Part model, mm, in its own coordinate system. A direction names the side the tool comes from. Coordinates: 2 decimals unless noted, no trailing zeros. Loops run counter-clockwise (first coordinate to the right, second up) from the corner with the lowest first, then second, coordinate; pieces in that order, holes last. Notation, with made-up numbers: (56.25, 14) - (72.25, 14) arc R12 cw to (72.25, 34) - close; hole circle Ø2 at (11, 3.25). An arc over 180 degrees is marked (long way). Answer as CSV lines item,"result".
from build123d import *

# Parameters (mm, degrees)
BOSS_EXTRUDE1_DEPTH      = 5
BOSS_EXTRUDE1_DEPTH_BACK = 5
SKETCH1_R                = 6.5
SKETCH1_R_2              = 4.5
SKETCH2_R                = 6.5
BOSS_EXTRUDE2_DEPTH      = 1
CUT_EXTRUDE1_START       = -8
CUT_EXTRUDE1_DEPTH       = 15
SKETCH6_W                = 4.3
SKETCH6_H                = 17.25833025
CUT_EXTRUDE2_DEPTH       = 10
CUT_EXTRUDE3_DEPTH       = 22.553121401
CUT_EXTRUDE3_DEPTH_BACK  = 22.553121401
SKETCH7_R                = 2
SKETCH8_W                = 9.14694849
SKETCH8_H                = 3.258330249
CUT_EXTRUDE4_DEPTH       = 7.682935
FILLET2_R                = 4
BOSS_EXTRUDE4_REACH      = 25.047
CUT_EXTRUDE5_DEPTH       = 19.647410958
CUT_EXTRUDE5_DEPTH_BACK  = 19.647410958
SKETCH10_R               = 2.1


with BuildPart() as part:
    # Sketch1 → Boss-Extrude1 (new, two sides: drawn at the far end of the back side and taken through both)
    with BuildSketch(Plane.XY.offset(-BOSS_EXTRUDE1_DEPTH_BACK)):
        Circle(SKETCH1_R)
        Circle(SKETCH1_R_2, mode=Mode.SUBTRACT)
    extrude(amount=BOSS_EXTRUDE1_DEPTH + BOSS_EXTRUDE1_DEPTH_BACK)

    # Sketch2 → Boss-Extrude2 (add)
    with BuildSketch(Plane.XY.offset(5)):
        Circle(SKETCH2_R)
    extrude(amount=BOSS_EXTRUDE2_DEPTH)

    # Sweep1: read off the stored shape, not the designer's step
    # Sweep1: loft between two sections, ruled curve by curve
    sweep1_from = [
        Edge.make_bspline([(6.5, 0, 6), (6.5, 13, 6), (-6.5, 13, 6), (-6.5, 0, 6), (-6.5, -13, 6), (6.5, -13, 6), (6.5, 0, 6)], [0, 0, 0, 0, 0.5, 0.5, 0.5, 1, 1, 1, 1], 3, [1, 0.333333333, 0.333333333, 1, 0.333333333, 0.333333333, 1]),
    ]
    sweep1_to = [
        Edge.make_bspline([(6.5, -7, 18.124355653), (6.5, 6, 18.124355653), (-6.5, 6, 18.124355653), (-6.5, -7, 18.124355653), (-6.5, -20, 18.124355653), (6.5, -20, 18.124355653), (6.5, -7, 18.124355653)], [0, 0, 0, 0, 0.5, 0.5, 0.5, 1, 1, 1, 1], 3, [1, 0.333333333, 0.333333333, 1, 0.333333333, 0.333333333, 1]),
    ]
    sweep1 = Solid(Shell([*[Face.make_surface_from_curves(sweep1_from[k], sweep1_to[k]) for k in range(1)], Face(Wire(sweep1_from)), Face(Wire(sweep1_to))]))
    add(sweep1)

    # Cut-Extrude1: read off the stored shape, not the designer's step
    # Cut-Extrude1 outline → Cut-Extrude1 (cut)
    with BuildSketch(Plane(origin=(0, 0, 0), x_dir=(0, 0, -1), z_dir=(1, 0, 0)).offset(CUT_EXTRUDE1_START)):
        Polygon((-12.495190528, -10.25), (-18.124355653, -0.5), (-18.124355653, -13.5), align=None)
    extrude(amount=CUT_EXTRUDE1_DEPTH, mode=Mode.SUBTRACT)

    # Sketch6 → Cut-Extrude2 (cut)
    with BuildSketch(Plane(origin=(0, -7.973076211, 13.809773091), x_dir=(1, 0, 0), z_dir=(0, -0.5000000000000006, 0.8660254037844384))):
        Rectangle(SKETCH6_W, SKETCH6_H)
    extrude(amount=-CUT_EXTRUDE2_DEPTH, mode=Mode.SUBTRACT)

    # Sketch7 → Cut-Extrude3 (cut, two sides: drawn at the far end of the back side and taken through both)
    with BuildSketch(Plane(origin=(0, 0, 0), x_dir=(0, 0, -1), z_dir=(1, 0, 0)).offset(-CUT_EXTRUDE3_DEPTH_BACK)):
        with Locations(Location((-11.845671476, -3.375, 0), (0, 0, 30))):
            Circle(SKETCH7_R)
    extrude(amount=CUT_EXTRUDE3_DEPTH + CUT_EXTRUDE3_DEPTH_BACK, mode=Mode.SUBTRACT)

    # Sketch8 → Cut-Extrude4 (cut)
    with BuildSketch(Plane(origin=(0, -7.973076211, 13.809773091), x_dir=(1, 0, 0), z_dir=(0, -0.5000000000000004, 0.8660254037844384))):
        with Locations((0, 8.629165125)):
            Rectangle(SKETCH8_W, SKETCH8_H)
        with Locations((0, -2.629165125)):
            Rectangle(SKETCH8_W, SKETCH8_H)
    extrude(amount=-CUT_EXTRUDE4_DEPTH, mode=Mode.SUBTRACT)

    # Fillet2
    # the kernel refuses this fillet: 4 mm, written as the material it takes off along each edge
    with BuildSketch(Plane(origin=(14.573474245, -1.910898385, 17.309773091), x_dir=(0, -0.8660254037646593, -0.5000000000342589), z_dir=(-1, 0, 0)), Plane(origin=(7.85, -1.910898385, 17.309773091), x_dir=(0, -0.8660254037646593, -0.5000000000342589), z_dir=(-1, 0, 0)), Plane(origin=(14.573474245, -8.839101615, 13.309773091), x_dir=(0, 0.5000000000000003, -0.8660254037844386), z_dir=(-1, 0, 0))) as fillet2_piece_1:
        with BuildLine():
            CenterArc((FILLET2_R, -FILLET2_R), FILLET2_R, 90, 90.000000002)
            Line((FILLET2_R * 3.95581923922e-11, -FILLET2_R), (0, 0))
            Line((0, 0), (FILLET2_R, 0))
        make_face()
    extrude(amount=22.423474245, mode=Mode.SUBTRACT)
    with BuildSketch(Plane(origin=(7.85, -8.839101615, 13.309773091), x_dir=(0, 0.8660254038042173, 0.49999999996574257), z_dir=(-1, 0, 0))) as fillet2_piece_2:
        with BuildLine():
            CenterArc((FILLET2_R, FILLET2_R), FILLET2_R, 179.999999998, 89.999999998)
            Line((FILLET2_R * 3.95576715485e-11, FILLET2_R), (0, 0))
            Line((0, 0), (FILLET2_R, 0))
        make_face()
    extrude(amount=22.423474245, mode=Mode.SUBTRACT)

    # Sketch9 → Boss-Extrude4 (add, up to next)
    with BuildSketch(Plane(origin=(0, 0, -5), x_dir=(-1, 0, 0), z_dir=(0, 0, -1)), mode=Mode.PRIVATE) as boss_extrude4_sk1:
        with BuildLine():
            Line((-3.15, 3.213642793), (-3.15, -3.213642793))
            ThreePointArc((-3.15, -3.213642793), (-4.5, 0), (-3.15, 3.213642793))
        make_face()
    boss_extrude4_tool1 = extrude(boss_extrude4_sk1.sketch, amount=-BOSS_EXTRUDE4_REACH, mode=Mode.PRIVATE) - part.part
    # Sketch9 → Boss-Extrude4 (add, up to next)
    with BuildSketch(Plane(origin=(0, 0, -5), x_dir=(-1, 0, 0), z_dir=(0, 0, -1)), mode=Mode.PRIVATE) as boss_extrude4_sk2:
        with BuildLine():
            Line((3.15, 3.213642793), (3.15, -3.213642793))
            ThreePointArc((3.15, -3.213642793), (4.5, 0), (3.15, 3.213642793))
        make_face()
    boss_extrude4_tool2 = extrude(boss_extrude4_sk2.sketch, amount=-BOSS_EXTRUDE4_REACH, mode=Mode.PRIVATE) - part.part
    add(boss_extrude4_tool1.solids().sort_by_distance((3.697607, 0, -5))[0])
    add(boss_extrude4_tool2.solids().sort_by_distance((-3.697607, 0, -5))[0])

    # Sketch10 → Cut-Extrude5 (cut, two sides: drawn at the far end of the back side and taken through both)
    with BuildSketch(Plane(origin=(0, 0, 0), x_dir=(0, 0, -1), z_dir=(1, 0, 0)).offset(-CUT_EXTRUDE5_DEPTH_BACK)):
        Circle(SKETCH10_R)
    extrude(amount=CUT_EXTRUDE5_DEPTH + CUT_EXTRUDE5_DEPTH_BACK, mode=Mode.SUBTRACT)


solid = part.part
Q1. Wall check: L1, parallel to X at y = -0.25, z = 4.25; L2, parallel to X at y = 0.75, z = 7.75; L3, parallel to Y at x = -0.75, z = 1. Give the ranges that are in metal, low to high.
Results:
L1,"x = -6.5 to -3.15, 3.15 to 6.5"
L2,"x = -6.26 to -2.15, 2.15 to 6.26"
L3,"y = -6.46 to -4.44, 4.44 to 6.46"
Q2. Saw through at A-A (z = 0). Give the cut face in (x, y).
Results:
outline,"(-6.15, -2.1) arc R6.5 ccw to (6.15, -2.1) - (3.15, -2.1) - (3.15, -3.21) arc R4.5 cw to (-3.15, -3.21) - (-3.15, -2.1) - close; (-6.15, 2.1) - (-3.15, 2.1) - (-3.15, 3.21) arc R4.5 cw to (3.15, 3.21) - (3.15, 2.1) - (6.15, 2.1) arc R6.5 ccw to start"
Q3. Flat gauge pins, fed straight in: pin 1 (1.5 mm diameter, centred on y = 1.5, z = 10.5, fed in from +X); pin 2 (5 mm diameter, centred on y = -3, z = 1.5, fed in from +X); pin 3 (3.5 mm diameter, centred on y = -3.38, z = 11.85, fed in from +X) (1 decimal); pin 4 (2 mm diameter, centred on y = -4, z = 4, fed in from -X). Where does each tip first touch, or does it go through?
Results:
pin 1,"stops at x = 5.64"
pin 2,"stops at x = 6.48"
pin 3,"passes through"
pin 4,"stops at x = -5.77"
Q4. Two-plate mould, pull along Y, no slides. Class faces 6 (the face through (-0.03, 0.688, 7.263)), 7 (the face through (4, 0, -5)), 8 (the face through (0, -4.5, -0.1)): released by +Y, released by -Y, zero draft, split by the parting line, or undercut.
Results:
face 6,"released by -Y"
face 7,"zero draft"
face 8,"undercut"
Q5. Saw through at B-B (y = -0.75). Count the separate pieces of the cut face and the enclosed holes in it, then the cut area to 3 significant figures.
Results:
separate pieces,"3"
enclosed holes,"0"
area,"124 mm^2"
Q6. Which spindle directions (+Z, -Z, +X, -X, +Y, -Y) get a long thin tool onto all of the face, cutting with end or side? Do faces 1 (the face through (3.075, 2.38, 10.916)), 2 (the face through (0, 4.5, -0.1)), 3 (the face through (-0.03, -5.492, 3.695)), 4 (the face through (-4.36, -4.3, 13.62)), 5 (the face through (-3.109, -5.432, 6.406)). Say none if no direction does.
Results:
face 1,"+Z, +X, -X"
face 2,"-Z"
face 3,"+Z, -Y"
face 4,"+X, -X"
face 5,"+X, -X, -Y"
